Check sheet for the modelled part. Datum: model origin and axes. Units: mm. A direction names the side the tool comes from. Coordinates: 2 decimals unless noted, no trailing zeros. Write each loop counter-clockwise with the first axis right and the second up, starting at its lowest first coordinate (ties: lowest second). Pieces come first, ordered by that corner, then holes. Notation, with made-up numbers: M -3.5,38.25 L 51.5,38.25 A24 ccw 51.5,48.25 Z; hole C 73.5,39.25 d10. An arc over 180 degrees is marked long. Answer as CSV lines item,"result". Start each with the question number.
1) Section check C-C (z = -5.25). Record the cut outline in (x, y).
2) Section check D-D (y = 2.5). Record the cut outline in (x, z) (3 decimals).
3) Access from +Z, -Z, +X, -X, +Y, -Y to the whole of each face (thin tool, end or side, straight path). Record for faces 5 (the flat face through (12, -23, -0.75)), 6 (the flat face through (13, -23, -10)), 7 (the flat face through (10.5, 23, -10)).
4) Material ranges on L1, parallel to Z at x = 12.05, y = 25; L2, parallel to X at y = 1, z = -15.5; L3, parallel to Y at x = 12.4, z = -15, recorded low to high. Write a range as [from, to].
5) Go/stop test with flat-tipped pins: pin 1 Ø2 at (y, z) = (2, -5) entering from +X; pin 2 Ø8 at (y, z) = (-20, -4.5) entering from +X; pin 3 Ø10 at (x, z) = (-1, -11) entering from +Y; pin 4 Ø4 at (x, z) = (11.5, -18) entering from +Y. Record where each tip stops, or that it passes through.
6) Section check B-B (x = 16). Record the cut outline in (y, z), and give its area (3 significant figures).
7) Section check A-A (y = 10.5). Record the cut outline in (x, z) (3 decimals).
8) Draft check along Y on faces 1 (the flat face through (12, -27, -10)), 2 (the cylindrical face through (11.77, -22.8, -15.08)), 3 (the cylindrical face through (11.77, -22.8, -5.08)), 4 (the flat face through (26, 11, -10)). Enter one of: +Y half, -Y half, draft (parallel to the pull), parting line (faces both ways), or undercut.
from build123d import *

# Parameters (mm, degrees)
SKETCH1_W           = 37
SKETCH1_H           = 40
BOSS_EXTRUDE1_DEPTH = 20
SKETCH2_W           = 18.5
SKETCH2_H           = 54
BOSS_EXTRUDE2_DEPTH = 2.5
FILLET1_R           = 1.5
CUT_EXTRUDE1_REACH  = 48.057
SKETCH3_R           = 2.2
SKETCH4_R           = 9.5
BOSS_EXTRUDE3_DEPTH = 2.2
SKETCH5_W           = 17.75
SKETCH5_H           = 23.804167323
BOSS_EXTRUDE4_DEPTH = 2.2
SKETCH6_R           = 6.65
BOSS_EXTRUDE5_DEPTH = 1.4
SKETCH7_R           = 2.925
BOSS_EXTRUDE6_DEPTH = 3.9


with BuildPart() as part:
    # Sketch1 → Boss-Extrude1 (new body)
    with BuildSketch(Plane.XY):
        Rectangle(SKETCH1_W, SKETCH1_H)
    extrude(amount=-BOSS_EXTRUDE1_DEPTH)

    # Sketch2 → Boss-Extrude2 (add)
    with BuildSketch(Plane.ZY.offset(-10.5)):
        with Locations((-10, 0)):
            Rectangle(SKETCH2_W, SKETCH2_H)
    extrude(amount=-BOSS_EXTRUDE2_DEPTH)

    # Fillet1
    fillet1_edges = [part.edges().sort_by_distance(p)[0] for p in [
        (11.75, -27, -19.25),
        (11.75, 27, -0.75),
        (11.75, -27, -0.75),
        (11.75, 27, -19.25),
    ]]
    fillet(fillet1_edges, radius=FILLET1_R)

    # Sketch3 → Cut-Extrude1 (cut, up to next)
    with BuildSketch(Plane(origin=(13, 0, 0), x_dir=(0, 0, -1), z_dir=(1, 0, 0)), mode=Mode.PRIVATE) as cut_extrude1_sk1:
        with Locations((5, 25)):
            Circle(SKETCH3_R)
    cut_extrude1_tool1 = extrude(cut_extrude1_sk1.sketch, amount=-CUT_EXTRUDE1_REACH, mode=Mode.PRIVATE) & part.part
    # Sketch3 → Cut-Extrude1 (cut, up to next)
    with BuildSketch(Plane(origin=(13, 0, 0), x_dir=(0, 0, -1), z_dir=(1, 0, 0)), mode=Mode.PRIVATE) as cut_extrude1_sk2:
        with Locations((15, 25)):
            Circle(SKETCH3_R)
    cut_extrude1_tool2 = extrude(cut_extrude1_sk2.sketch, amount=-CUT_EXTRUDE1_REACH, mode=Mode.PRIVATE) & part.part
    # Sketch3 → Cut-Extrude1 (cut, up to next)
    with BuildSketch(Plane(origin=(13, 0, 0), x_dir=(0, 0, -1), z_dir=(1, 0, 0)), mode=Mode.PRIVATE) as cut_extrude1_sk3:
        with Locations((5, -25)):
            Circle(SKETCH3_R)
    cut_extrude1_tool3 = extrude(cut_extrude1_sk3.sketch, amount=-CUT_EXTRUDE1_REACH, mode=Mode.PRIVATE) & part.part
    # Sketch3 → Cut-Extrude1 (cut, up to next)
    with BuildSketch(Plane(origin=(13, 0, 0), x_dir=(0, 0, -1), z_dir=(1, 0, 0)), mode=Mode.PRIVATE) as cut_extrude1_sk4:
        with Locations((15, -25)):
            Circle(SKETCH3_R)
    cut_extrude1_tool4 = extrude(cut_extrude1_sk4.sketch, amount=-CUT_EXTRUDE1_REACH, mode=Mode.PRIVATE) & part.part
    add(cut_extrude1_tool1.solids().sort_by_distance((13, 25, -5))[0], mode=Mode.SUBTRACT)
    add(cut_extrude1_tool2.solids().sort_by_distance((13, 25, -15))[0], mode=Mode.SUBTRACT)
    add(cut_extrude1_tool3.solids().sort_by_distance((13, -25, -5))[0], mode=Mode.SUBTRACT)
    add(cut_extrude1_tool4.solids().sort_by_distance((13, -25, -15))[0], mode=Mode.SUBTRACT)

    # Sketch4 → Boss-Extrude3 (add)
    with BuildSketch(Plane(origin=(18.5, 0, 0), x_dir=(0, 0, -1), z_dir=(1, 0, 0))):
        with Locations(Location((10, 10.5, 0), (0, 0, 90))):
            Circle(SKETCH4_R)
    extrude(amount=BOSS_EXTRUDE3_DEPTH)

    # Sketch5 → Boss-Extrude4 (add)
    with BuildSketch(Plane(origin=(18.5, 0, 0), x_dir=(0, 0, -1), z_dir=(1, 0, 0))):
        with Locations((10, -1.797916339)):
            Rectangle(SKETCH5_W, SKETCH5_H)
    extrude(amount=BOSS_EXTRUDE4_DEPTH)

    # Sketch6 → Boss-Extrude5 (add)
    with BuildSketch(Plane(origin=(20.7, 0, 0), x_dir=(0, 0, -1), z_dir=(1, 0, 0))):
        with Locations((10, 10.5)):
            Circle(SKETCH6_R)
    extrude(amount=BOSS_EXTRUDE5_DEPTH)

    # Sketch7 → Boss-Extrude6 (add)
    with BuildSketch(Plane(origin=(22.1, 0, 0), x_dir=(0, 0, -1), z_dir=(1, 0, 0))):
        with Locations((10, 10.5)):
            Circle(SKETCH7_R)
    extrude(amount=BOSS_EXTRUDE6_DEPTH)


solid = part.part
Results found:
1,outline,"M -18.5,-20 L 10.5,-20 L 10.5,-22.81 L 13,-22.81 L 13,-20 L 18.5,-20 L 18.5,-13.7 L 20.7,-13.7 L 20.7,5.85 L 22.1,5.85 L 22.1,15.15 L 20.7,15.15 L 20.7,18.73 L 18.5,18.73 L 18.5,20 L 13,20 L 13,22.81 L 10.5,22.81 L 10.5,20 L -18.5,20 Z"
2,outline,"M -18.5,-20 L 18.5,-20 L 18.5,-18.875 L 20.7,-18.875 L 20.7,-1.125 L 18.5,-1.125 L 18.5,0 L -18.5,0 Z"
3,face 5,"+Z, +X, -X, -Y"
3,face 6,"+Z, -Z, +X, -Y"
3,face 7,"+Z, -Z, -X, +Y"
4,L1,"z = [-19.25, -17.2], [-12.8, -7.2], [-2.8, -0.75]"
4,L2,"x = [-18.5, 20.7]"
4,L3,"y = [-22.8, 22.8]"
5,pin 1,"stops at x = 20.7"
5,pin 2,"stops at x = 18.5"
5,pin 3,"stops at y = 20"
5,pin 4,"stops at y = 27"
6,outline,"M -20,-20 L 20,-20 L 20,0 L -20,0 Z"
6,area,"800 mm2"
7,outline,"M -18.5,-20 L 18.5,-20 L 18.5,-19.5 L 20.7,-19.5 L 20.7,-16.65 L 22.1,-16.65 L 22.1,-12.925 L 26,-12.925 L 26,-7.075 L 22.1,-7.075 L 22.1,-3.35 L 20.7,-3.35 L 20.7,-0.5 L 18.5,-0.5 L 18.5,0 L -18.5,0 Z"
8,face 1,"-Y half"
8,face 2,"undercut"
8,face 3,"undercut"
8,face 4,"draft"
